Geometry: final body of the model. Coordinates: model frame, mm. Face numbers are marked on the shaded views. A direction names the side the tool comes from. Round coordinates to 2 decimals unless told otherwise and drop trailing zeros. Write each loop counter-clockwise with the first axis right and the second up, starting at its lowest first coordinate (ties: lowest second). Pieces come first, ordered by that corner, then holes.
from build123d import *

# Parameters (mm, degrees)
F0_R      = 23.135211
F1_DEPTH  = 25.4
F2_R      = 26.447922
F2_R_2    = 23.135211
F1_FACE_R = 23.135211
F3_DEPTH  = 25.4
F4_R      = 5.08


with BuildPart() as f1:
    # F0 (on Top) → F1 (new body)
    with BuildSketch(Plane.XY):
        Circle(F0_R)
    extrude(amount=F1_DEPTH)

    # F2 (on face) + F1_face (on face) → F3 (join)
    with BuildSketch(Plane.XY.offset(25.4)):
        Circle(F2_R)
        Circle(F2_R_2, mode=Mode.SUBTRACT)
        Circle(F2_R_2)
    with BuildSketch(Plane.XY.offset(25.4)):
        Circle(F1_FACE_R)
    extrude(amount=F3_DEPTH)

    # F4
    f4_edges = [f1.edges().sort_by_distance(p)[0] for p in [
        (-26.447922, 0, 50.8),
    ]]
    fillet(f4_edges, radius=F4_R)


solid = f1.part
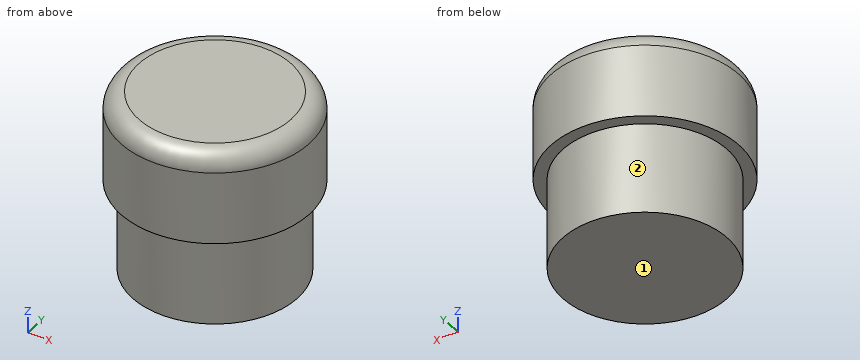
1) Reachability of the marked faces 1 and 2 from +Z, -Z, +X, -X, +Y, -Y: full face, straight path, thin tool, end or side. Return the list, or none.
2) Section D-D on z = 30. Output: boundary loops of the cut face in (x, y).
3) Section A-A on x = 0. Output: boundary loops of the cut face in (y, z), plus the area to 3 significant figures.
4) Section C-C on z = 18. Output: boundary loops of the cut face in (x, y).
5) First-contact query: P1, Ø3, axis at x = -14, y = 12.5, coming from the -Z side; P2, Ø1, axis at y = 2, z = 8.5, coming from the +X side; P3, Ø10, axis at x = 7, z = 32.5, coming from the +Y side; P4, Ø1.5, axis at x = -9, z = 7, coming from the -Y side. Flat tips, straight axial feed; report the tip coordinate or a pass-through.
6) Line query: probe 1 along X at (y, z) = (18, 23.5); probe 2 along Y at (x, z) = (-8, 4.5); probe 3 along X at (y, z) = (17, 37). Output: solid intervals per line, ascending.
Filled in:
1. face 1: -Z, +X, -X, +Y, -Y
1. face 2: -Z
2. outline: circle Ø52.9 at (0, 0)
3. outline: (-26.45, 25.4) - (-23.14, 25.4) - (-23.14, 0) - (23.14, 0) - (23.14, 25.4) - (26.45, 25.4) - (26.45, 45.72) arc R5.08 ccw to (21.37, 50.8) - (-21.37, 50.8) arc R5.08 ccw to (-26.45, 45.72) - close
3. area: 2,510 mm2
4. outline: circle Ø46.27 at (0, 0)
5. P1: stops at z = 0
5. P2: stops at x = 23.09
5. P3: stops at y = 26.37
5. P4: stops at y = -21.61
6. probe 1: x = -14.53 to 14.53
6. probe 2: y = -21.71 to 21.71
6. probe 3: x = -20.26 to 20.26
